Geometry check sheet. Reference: the model listing, model coordinates, mm. A direction names the side the tool comes from. Coordinates: 2 decimals unless noted, no trailing zeros. Write each loop counter-clockwise with the first axis right and the second up, starting at its lowest first coordinate (ties: lowest second). Pieces come first, ordered by that corner, then holes. Notation, with made-up numbers: (-19, 74) -> (-1, 74) arc R13 cw to (-1, 91) -> close; hole circle Ø7 at (73.5, -10.75). An arc over 180 degrees is marked (long way). One line per question, with ' | ' between items.
from build123d import *

# Parameters (mm, degrees)
SKIZZE1_W                       = 5
SKIZZE1_H                       = 5
AUFSATZ_LINEAR_AUSTRAGEN1_DEPTH = 15
SKIZZE2_R                       = 1.25
SKIZZE2_R_2                     = 1.5
SCHNITT_LINEAR_AUSTRAGEN1_DEPTH = 9
SKIZZE3_R                       = 1.5
SCHNITT_LINEAR_AUSTRAGEN2_DEPTH = 9


with BuildPart() as part:
    # Skizze1 → Aufsatz-Linear austragen1 (new body)
    with BuildSketch(Plane.XY):
        Polygon((-7.5, -2.5), (-1.5, -2.5), (2.5, -2.5), (2.5, 2.5), (-7.5, 2.5), align=None)
        with Locations((5, 0)):
            Rectangle(SKIZZE1_W, SKIZZE1_H)
        Polygon((2.5, -2.5), (-1.5, -2.5), (2.5, -14), align=None)
        Polygon((2.5, -2.5), (2.5, -14), (2.5, -20), (7.5, -20), (7.5, -2.5), align=None)
    extrude(amount=AUFSATZ_LINEAR_AUSTRAGEN1_DEPTH)

    # Skizze2 → Schnitt-Linear austragen1 (cut)
    with BuildSketch(Plane(origin=(7.5, 0, 0), x_dir=(0, 0, -1), z_dir=(1, 0, 0))):
        with Locations(Location((-7.5, 0.45, 0), (0, 0, 90))):
            Circle(SKIZZE2_R)
        with Locations(Location((-7.5, -17.7, 0), (0, 0, 90))):
            Circle(SKIZZE2_R_2)
    extrude(amount=-SCHNITT_LINEAR_AUSTRAGEN1_DEPTH, mode=Mode.SUBTRACT)

    # Skizze3 → Schnitt-Linear austragen2 (cut)
    with BuildSketch(Plane.XZ.offset(2.5)):
        with Locations(Location((-4.5, 7.5, 0), (0, 0, 270))):
            Circle(SKIZZE3_R)
    extrude(amount=-SCHNITT_LINEAR_AUSTRAGEN2_DEPTH, mode=Mode.SUBTRACT)


solid = part.part
1. Cross-section at D-D on z = 7.5. Record the boundary of the cut face in (x, y).
Worked answers:
outline: (-7.5, -2.5) -> (-6, -2.5) -> (-6, 2.5) -> (-7.5, 2.5) -> close; (-3, -2.5) -> (-1.5, -2.5) -> (2.5, -14) -> (2.5, -16.2) -> (7.5, -16.2) -> (7.5, -0.8) -> (-1.5, -0.8) -> (-1.5, 1.7) -> (7.5, 1.7) -> (7.5, 2.5) -> (-3, 2.5) -> close; (2.5, -20) -> (7.5, -20) -> (7.5, -19.2) -> (2.5, -19.2) -> close
2. Tool access check on faces 5 (the face through (-4.5, -2.5, 5.7)), 6 (the face through (-1.5, 0, 8)), 7 (the face through (7.5, -9, 7)). Record the directions out of +Z, -Z, +X, -X, +Y, -Y that give a thin tool (end or side, any length) a straight path to the whole face; none if there is none.
Worked answers:
face 5: +Z, -Z, -X, -Y | face 6: +X | face 7: +Z, -Z, +X, +Y, -Y
3. Mould release check, pull along Z, two halves, no side actions. Record for faces 1 (the face through (2, -6, 0)), 2 (the face through (5.035, -16.314, 6.925)), 3 (the face through (3.06, 0.18, 6.28)), 4 (the face through (2.5, -16, 7)): released by +Z, released by -Z, zero draft, split by the parting line, or undercut.
Worked answers:
face 1: released by -Z | face 2: undercut | face 3: undercut | face 4: zero draft
4. Go/stop test with flat-tipped pins: P1, Ø1.5, axis at y = 0.45, z = 7.5, coming from the +X side; P2, Ø3, axis at y = -17.5, z = 5.5, coming from the -X side; P3, Ø1.5, axis at y = -9, z = 12.5, coming from the -X side; P4, Ø1.8, axis at x = -4.5, z = 7.5, coming from the +Y side. Record where each tip stops, or that it passes through.
Worked answers:
P1: x = -1.5 | P2: x = 2.5 | P3: x = 0.5 | P4: through
5. Cross-section at C-C on y = 0.45. Record the boundary of the cut face in (x, z), and give its area (3 significant figures).
Worked answers:
outline: (-7.5, 0) -> (7.5, 0) -> (7.5, 6.25) -> (-1.5, 6.25) -> (-1.5, 8.75) -> (7.5, 8.75) -> (7.5, 15) -> (-7.5, 15) -> close; hole circle Ø3 at (-4.5, 7.5) | area: 195 mm²
6. Cross-section at B-B on y = -17.7. Record the boundary of the cut face in (x, z).
Worked answers:
outline: (2.5, 0) -> (7.5, 0) -> (7.5, 6) -> (2.5, 6) -> close; (2.5, 9) -> (7.5, 9) -> (7.5, 15) -> (2.5, 15) -> close
7. Material ranges on line 1 (Z direction, x = 4.55, y = -17.7); line 2 (X direction, y = 0.75, z = 7.5); line 3 (Y direction, x = 4.5, z = 6.5), recorded low to high. Write a range as from..to.
Worked answers:
line 1: 0..6, 9..15 | line 2: -7.5..-6, -3..-1.5 | line 3: -20..-18.82, -16.58..-0.3, 1.2..2.5
8. Cross-section at A-A on x = -4.5. Record the boundary of the cut face in (y, z), and give its area (3 significant figures).
Worked answers:
outline: (-2.5, 0) -> (2.5, 0) -> (2.5, 6) -> (-2.5, 6) -> close; (-2.5, 9) -> (2.5, 9) -> (2.5, 15) -> (-2.5, 15) -> close | area: 60.0 mm²
